Design review of the part built by this model. Coordinates are the model's own, in mm. Coordinates: 2 decimals unless noted, no trailing zeros. Write each loop counter-clockwise with the first axis right and the second up, starting at its lowest first coordinate (ties: lowest second). Pieces come first, ordered by that corner, then holes.
Q1. Add section B-B, the plane z = -100. Give the boundary of the cut face in (x, y), plus the area to 3 significant figures.
Q2. Add section C-C, the plane y = 2.65. Give the boundary of the cut face in (x, z), plus the area to 3 significant figures.
Q3. Add section D-D, the plane x = 30.5. Give the boundary of the cut face in (y, z).
Q4. Clearance check with flat-ended pins moving along their axes: pin 1 Ø5 at (x, z) = (4, -75) entering from +Y; pin 2 Ø1 at (y, z) = (3, -101) entering from +X; pin 3 Ø1 at (y, z) = (0.5, -95) entering from -X. State where each tip first meets the part, or that it passes through.
Q5. Add section A-A, the plane x = 13.5. Give the boundary of the cut face in (y, z), plus the area to 3 significant figures.
Q6. To check wall thickness, follow probe 1 along Y at (x, z) = (20.5, -35); probe 2 along Y at (x, z) = (19, -88.5); probe 3 along Z at (x, y) = (21, 3.2). State the ranges of each line that lie inside material, in increasing order.
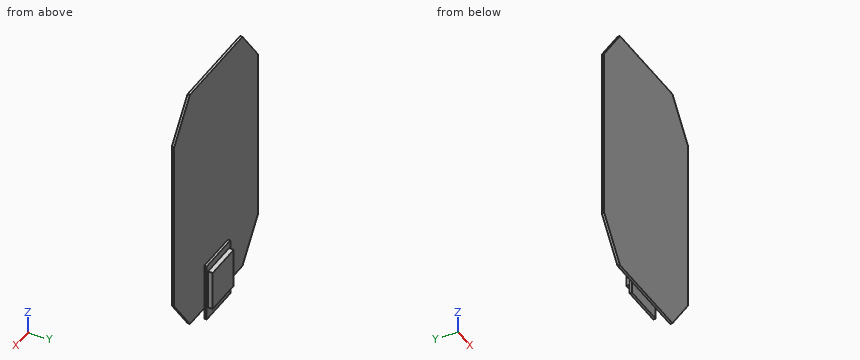
from build123d import *

# Parameters (mm, degrees)
BOSS_EXTRUDE3_DEPTH = 1
SKETCH5_W           = 8
SKETCH5_H           = 17
BOSS_EXTRUDE4_DEPTH = 3
SKETCH6_W           = 18
SKETCH6_H           = 25
BOSS_EXTRUDE5_DEPTH = 1
SKETCH7_W           = 18
SKETCH7_H           = 5.023609272
CUT_EXTRUDE4_DEPTH  = 1


with BuildPart() as part:
    # Sketch1 → Boss-Extrude3 (new body)
    with BuildSketch(Plane(origin=(0, 0, 0), x_dir=(1, 0, 0), z_dir=(0, 1, 0))):
        Polygon((-12, 54), (20, 54), (20, 108), (11, 108), (0, 108), (-12, 91.5), align=None)
        Polygon((20, 108), (20, 54), (52, 54), (52, 91.5), (40, 108), (29, 108), align=None)
        Polygon((-12, 16.5), (0, 0), (20, 0), (20, 54), (-12, 54), align=None)
        Polygon((20, 54), (20, 0), (40, 0), (52, 16.5), (52, 54), align=None)
        Polygon((11, 108), (20, 108), (29, 108), (29, 113.023609272), (11, 113.023609272), align=None)
    extrude(amount=BOSS_EXTRUDE3_DEPTH)

    # Sketch5 → Boss-Extrude4 (add)
    with BuildSketch(Plane(origin=(0, 1, 0), x_dir=(1, 0, 0), z_dir=(0, 1, 0))):
        with Locations((16, 99.523609272)):
            Rectangle(SKETCH5_W, SKETCH5_H)
        with Locations((24, 99.523609272)):
            Rectangle(SKETCH5_W, SKETCH5_H)
    extrude(amount=BOSS_EXTRUDE4_DEPTH)

    # Sketch6 → Boss-Extrude5 (add)
    with BuildSketch(Plane(origin=(0, 1, 0), x_dir=(1, 0, 0), z_dir=(0, 1, 0))):
        with Locations((20, 100.523609272)):
            Rectangle(SKETCH6_W, SKETCH6_H)
    extrude(amount=BOSS_EXTRUDE5_DEPTH)

    # Sketch7 → Cut-Extrude4 (cut)
    with BuildSketch(Plane.XZ):
        with Locations((20, -110.511804636)):
            Rectangle(SKETCH7_W, SKETCH7_H)
    extrude(amount=-CUT_EXTRUDE4_DEPTH, mode=Mode.SUBTRACT)


solid = part.part
Here are the results:
1. outline: (-5.82, 0) - (45.82, 0) - (45.82, 1) - (29, 1) - (29, 2) - (28, 2) - (28, 4) - (12, 4) - (12, 2) - (11, 2) - (11, 1) - (-5.82, 1) - close
1. area: 102 mm2
2. outline: (12, -108.02) - (28, -108.02) - (28, -91.02) - (12, -91.02) - close
2. area: 272 mm2
3. outline: (0, -108) - (1, -108) - (1, 0) - (0, 0) - close
4. pin 1: stops at y = 1
4. pin 2: stops at x = 28
4. pin 3: stops at x = -9.82
5. outline: (0, -108) - (1, -108) - (1, -113.02) - (2, -113.02) - (2, -108.02) - (4, -108.02) - (4, -91.02) - (2, -91.02) - (2, -88.02) - (1, -88.02) - (1, 0) - (0, 0) - close
5. area: 167 mm2
6. probe 1: y = 0 to 1
6. probe 2: y = 0 to 2
6. probe 3: z = -108.02 to -91.02
